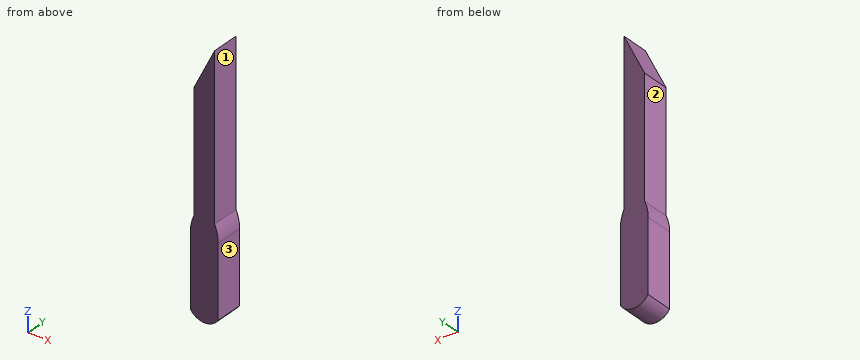
from build123d import *

# Parameters (mm, degrees)
F1_DEPTH    = 3.5
F2_T1_DEPTH = 13.6927447268
F2_T3_DEPTH = 13.6880389421


# Not quite as in the source:
# - a fillet or chamfer that OpenCascade refuses, or shapes differently, is made with other operations: its cross-section is extruded or revolved along the edge and cut away or added


with BuildPart() as f1:
    # F0 (on Front) → F1 (new body)
    with BuildSketch(Plane.XZ):
        with BuildLine():
            Line((-12.9772726037, -35.7954576612), (-16.4772726037, -35.7954576612))
            ThreePointArc((-16.4772726037, -35.7954576612), (-14.7272726037, -36.734376134), (-12.9772726037, -35.7954576612))
        make_face()
        Polygon((-16.0428304225, -9.6928073466), (-16.0428304225, -24.6928073466), (-13.4112946689, -24.6928073466), (-13.4112946689, -4.3468838558), align=None)
        Polygon((-16.4772726037, -24.6928073466), (-16.4772726037, -35.7954576612), (-12.9772726037, -35.7954576612), (-12.9772726037, -24.6928073466), (-13.4112946689, -24.6928073466), (-16.0428304225, -24.6928073466), align=None)
    extrude(amount=F1_DEPTH)

    # F2: fillet of radius 5 on 2 edges, made by hand

    # F2_s2 → F2_t1 (cut)
    with BuildSketch(Plane.XZ.offset(-5.0963723634)):
        with BuildLine():
            ThreePointArc((-16.0428304225, -24.6928073466), (-16.3674560917, -25.6891924599), (-16.4772726037, -26.7313562919))
            Line((-16.4772726037, -26.7313562919), (-16.4772726037, -24.6928073466))
            Line((-16.4772726037, -24.6928073466), (-16.0428304225, -24.6928073466))
        make_face()
    extrude(amount=F2_T1_DEPTH, mode=Mode.SUBTRACT)

    # F2_s4 → F2_t3 (cut)
    with BuildSketch(Plane.XZ.offset(-5.094019471)):
        with BuildLine():
            ThreePointArc((-12.9772726037, -26.730415135), (-13.0869817292, -25.6887553234), (-13.4112946689, -24.6928073466))
            Line((-13.4112946689, -24.6928073466), (-12.9772726037, -24.6928073466))
            Line((-12.9772726037, -24.6928073466), (-12.9772726037, -26.730415135))
        make_face()
    extrude(amount=F2_T3_DEPTH, mode=Mode.SUBTRACT)


solid = f1.part
Source: CAD feature listing. Evaluate the final solid. Frame: model axes, mm. Face numbers are marked on the shaded views. A direction names the side the tool comes from. Round coordinates to 2 decimals unless told otherwise and drop trailing zeros. Loops run counter-clockwise (first coordinate to the right, second up) from the corner with the lowest first, then second, coordinate; pieces in that order, holes last. Notation, with made-up numbers: (63.25, 18) - (89.25, 18) arc R25 cw to (89.25, 57) - close; hole circle Ø9 at (3.5, 8.5). An arc over 180 degrees is marked (long way). Write item = value, one per line. Start each with the question number.
Item 1: Section query B-B on z = -18. Output: boundary loops of the cut face in (x, y), plus the area to 3 significant figures.
Item 2: First-contact query: pin 1 Ø1.5 at (x, y) = (-14, -1.5) entering from -Z; pin 2 Ø1.8 at (y, z) = (-1.5, -20) entering from -X; pin 3 Ø1.8 at (y, z) = (-2.5, -10) entering from +X. Flat tips, straight axial feed; report the tip coordinate or a pass-through.
Item 3: Section query C-C on x = -14.15. Output: boundary loops of the cut face in (y, z), plus the area to 3 significant figures.
Item 4: Section query A-A on y = -3.1. Output: boundary loops of the cut face in (x, z), plus the area to 3 significant figures.
Item 5: Reachability of the marked faces 1, 2 and 3 from +Z, -Z, +X, -X, +Y, -Y: full face, straight path, thin tool, end or side. Return the list, or none.
Item 6: Material intervals for line 1 (X direction, y = -0.25, z = -16); line 2 (Z direction, x = -15.35, y = -1.95); line 3 (Z direction, x = -14, y = -2.3), sorted ascending.
Results list:
q1.outline = (-16.04, -3.5) - (-13.41, -3.5) - (-13.41, 0) - (-16.04, 0) - close
q1.area = 9.21 mm²
q2.pin_1 = -36.73
q2.pin_2 = -16.04
q2.pin_3 = -13.41
q3.outline = (-3.5, -36.65) - (0, -36.65) - (0, -5.85) - (-3.5, -5.85) - close
q3.area = 108 mm²
q4.outline = (-16.48, -35.8) arc R2.1 ccw to (-12.98, -35.8) - (-12.98, -26.73) arc R5 ccw to (-13.41, -24.69) - (-13.41, -4.35) - (-16.04, -9.69) - (-16.04, -24.69) arc R5 ccw to (-16.48, -26.73) - close
q4.area = 87.1 mm²
q5.face_1 = +Z, +X, +Y, -Y
q5.face_2 = +Z, -X, +Y, -Y
q5.face_3 = +Z, -Z, +X, +Y, -Y
q6.line_1 = -16.04 to -13.41
q6.line_2 = -36.64 to -8.29
q6.line_3 = -36.6 to -5.54
